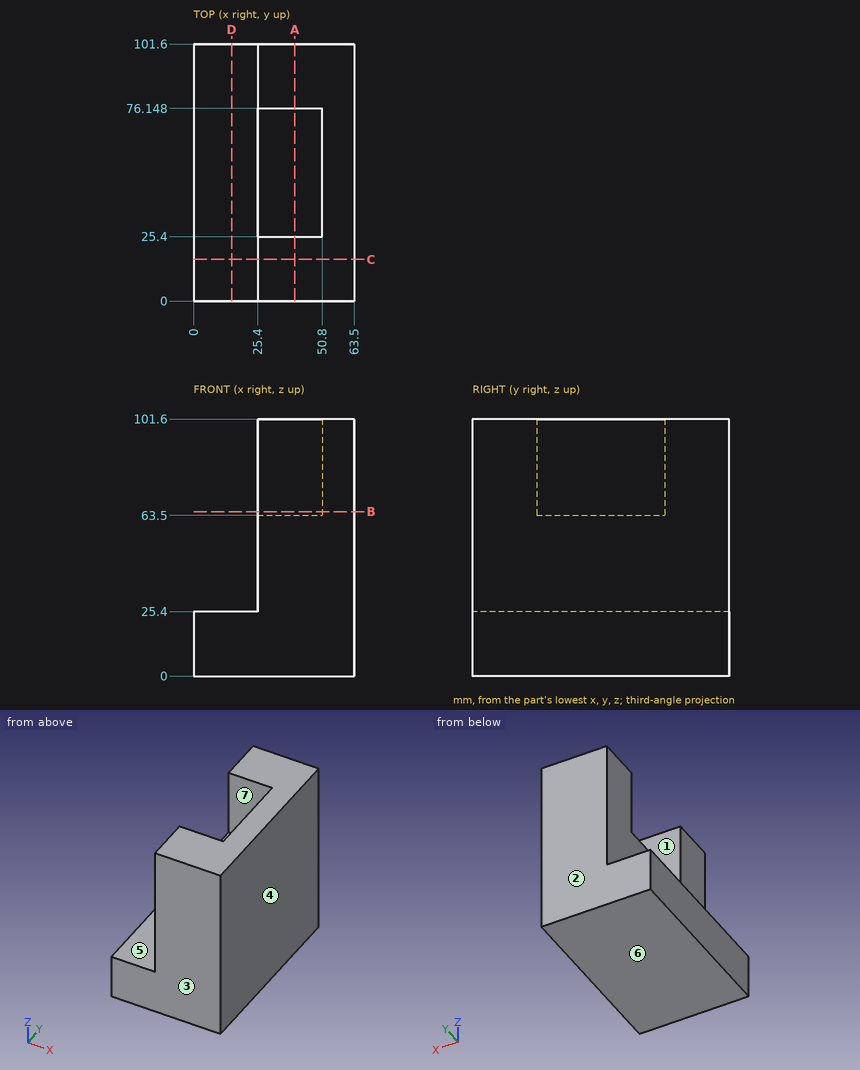
Job drawing, mm, ordinate dimensions from the low corner. One solid piece. A direction names the side the tool comes from. Round coordinates to 2 decimals unless told otherwise and drop trailing zeros. Write each loop counter-clockwise with the first axis right and the second up, starting at its lowest first coordinate (ties: lowest second). Pieces come first, ordered by that corner, then holes. Notation, with made-up numbers: M 3.25,-10 L 60.25,-10 A28 cw 60.25,8 Z; hole C 38.25,-7.75 d6. An arc over 180 degrees is marked long. Return JSON: item names as keys, results as strings. Group by question number.
(1) Drill centre lines: probe 1 along Z at (x, y) = (4.5, 88.5); probe 2 along X at (y, z) = (86, 87); probe 3 along Z at (x, y) = (33, 66). Where is each one in solid material? Low to high.
(2) Pin check, flat tips, straight feed: pin 1 Ø12.5 at (x, y) = (34.5, 44.5) entering from +Z; pin 2 Ø10 at (y, z) = (48.5, 45.5) entering from -X; pin 3 Ø19 at (y, z) = (49, 89.5) entering from -X. Stop position of each tip, or through.
(3) Saw through at C-C on y = 16.5. Write the cut outline in (x, z).
(4) Saw through at A-A on x = 40. Write the cut outline in (y, z).
(5) Saw through at B-B on z = 65. Write the cut outline in (x, y).
(6) Two-plate mould, pull along Y, no slides. Class the marked faces 1, 2, 3 and 4: +Y half, -Y half, draft (parallel to the pull), parting line (faces both ways), or undercut.
(7) Which spindle directions (+Z, -Z, +X, -X, +Y, -Y) get a long thin tool onto all of the face, cutting with end or side? Do the marked faces 5, 6 and 7. Say none if no direction does.
(8) Saw through at D-D on x = 15. Write the cut outline in (y, z), then the cut area to 3 significant figures.
Returned:
{
 "1": {"probe 1": "0 to 25.4", "probe 2": "25.4 to 63.5", "probe 3": "0 to 63.5"},
 "2": {"pin 1": "z = 63.5", "pin 2": "x = 25.4", "pin 3": "x = 50.8"},
 "3": {"outline": "M 0,0 L 63.5,0 L 63.5,101.6 L 25.4,101.6 L 25.4,25.4 L 0,25.4 Z"},
 "4": {"outline": "M 0,0 L 101.6,0 L 101.6,101.6 L 76.15,101.6 L 76.15,63.5 L 25.4,63.5 L 25.4,101.6 L 0,101.6 Z"},
 "5": {"outline": "M 25.4,0 L 63.5,0 L 63.5,101.6 L 25.4,101.6 L 25.4,76.15 L 50.8,76.15 L 50.8,25.4 L 25.4,25.4 Z"},
 "6": {"face 1": "undercut", "face 2": "+Y half", "face 3": "-Y half", "face 4": "draft"},
 "7": {"face 5": "+Z, -X, +Y, -Y", "face 6": "-Z, +X, -X, +Y, -Y", "face 7": "+Z, -X"},
 "8": {"outline": "M 0,0 L 101.6,0 L 101.6,25.4 L 0,25.4 Z", "area": "2,580 mm²"}
}
